```python
from build123d import *

# Parameters (mm, degrees)
SKETCH1_W           = 50
SKETCH1_H           = 20
SKETCH1_R           = 2.75
BOSS_EXTRUDE1_DEPTH = 4
SKETCH2_R           = 5
BOSS_EXTRUDE2_DEPTH = 50
SKETCH3_R           = 6
BOSS_EXTRUDE3_DEPTH = 2


with BuildPart() as part:
    # Sketch1 → Boss-Extrude1 (new body)
    with BuildSketch(Plane.XY):
        Rectangle(SKETCH1_W, SKETCH1_H)
        with Locations((15, 0)):
            Circle(SKETCH1_R, mode=Mode.SUBTRACT)
        with Locations((-15, 0)):
            Circle(SKETCH1_R, mode=Mode.SUBTRACT)
    extrude(amount=-BOSS_EXTRUDE1_DEPTH)

    # Sketch2 → Boss-Extrude2 (add)
    with BuildSketch(Plane.XY):
        Circle(SKETCH2_R)
    extrude(amount=BOSS_EXTRUDE2_DEPTH)

    # Sketch3 → Boss-Extrude3 (add)
    with BuildSketch(Plane.XY.offset(50)):
        Circle(SKETCH3_R)
    extrude(amount=BOSS_EXTRUDE3_DEPTH)


solid = part.part
```
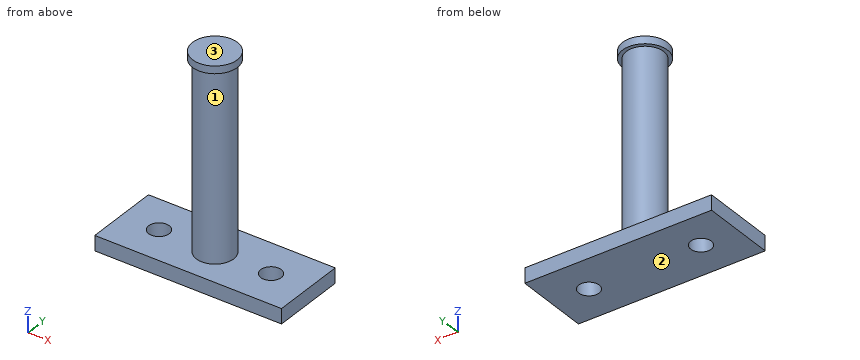
Geometry check sheet. Reference: the model listing, model coordinates, mm. Face numbers are marked on the shaded views. Give positions to 0.01 mm unless a question says otherwise; leave off trailing zeros. Write each loop counter-clockwise with the first axis right and the second up, starting at its lowest first coordinate (ties: lowest second). Pieces come first, ordered by that corner, then holes.
1) Section check A-A, the plane x = 15. Record the boundary of the cut face in (y, z), and give its area (3 significant figures).
2) Material ranges on L1, parallel to Z at x = 1, y = -5.25; L2, parallel to Y at x = -15, z = -1; L3, parallel to Z at x = 15.5, y = 8, recorded low to high.
3) Gauge pin test, flat ends, axial feed: pin 1 (1.5 mm diameter, centred on x = 15.5, y = -4, fed in from +Z); pin 2 (6 mm diameter, centred on y = 3.5, z = 14, fed in from +X); pin 3 (10 mm diameter, centred on y = 2.5, z = 38.5, fed in from -X). Record the tip position at first contact, or that the pin passes through.
4) Section check C-C, the plane x = 0. Record the boundary of the cut face in (y, z).
5) Section check D-D, the plane y = 6.75. Record the boundary of the cut face in (x, z).
6) Section check B-B, the plane y = 0. Record the boundary of the cut face in (x, z), and give its area (3 significant figures).
7) Release check for a two-part mould opening along Z. For the marked faces 1, 2 and 3 record: pulls with the +Z half, pulls with the -Z half, needs draft (parallel to the pull), parting line crosses it, or undercut.
Computed:
1. outline: (-10, -4) - (-2.75, -4) - (-2.75, 0) - (-10, 0) - close; (2.75, -4) - (10, -4) - (10, 0) - (2.75, 0) - close
1. area: 58.0 mm2
2. L1: z = -4 to 0, 50 to 52
2. L2: y = -10 to -2.75, 2.75 to 10
2. L3: z = -4 to 0
3. pin 1: stops at z = 0
3. pin 2: stops at x = 4.97
3. pin 3: stops at x = -5
4. outline: (-10, -4) - (10, -4) - (10, 0) - (5, 0) - (5, 50) - (6, 50) - (6, 52) - (-6, 52) - (-6, 50) - (-5, 50) - (-5, 0) - (-10, 0) - close
5. outline: (-25, -4) - (25, -4) - (25, 0) - (-25, 0) - close
6. outline: (-25, -4) - (-17.75, -4) - (-17.75, 0) - (-25, 0) - close; (-12.25, -4) - (12.25, -4) - (12.25, 0) - (5, 0) - (5, 50) - (6, 50) - (6, 52) - (-6, 52) - (-6, 50) - (-5, 50) - (-5, 0) - (-12.25, 0) - close; (17.75, -4) - (25, -4) - (25, 0) - (17.75, 0) - close
6. area: 680 mm2
7. face 1: undercut
7. face 2: pulls with the -Z half
7. face 3: pulls with the +Z half
